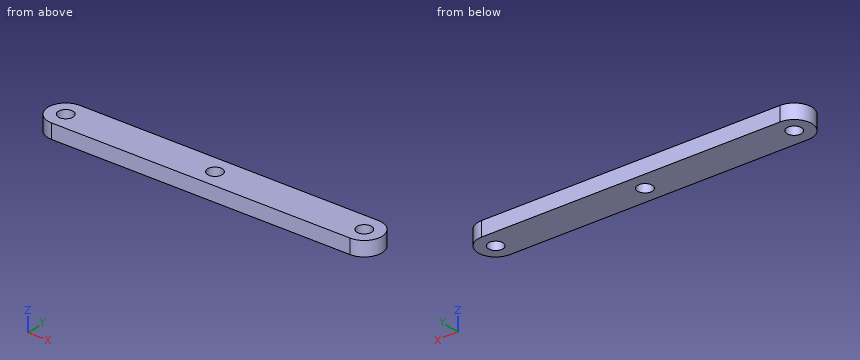
```python
from build123d import *

# Parameters (mm, degrees)
SKETCH1_R           = 2.5
BOSS_EXTRUDE1_DEPTH = 2.5


with BuildPart() as part:
    # Sketch1 → Boss-Extrude1 (new, symmetric)
    with BuildSketch(Plane.XY):
        with BuildLine():
            Line((-50, 6), (50, 6))
            ThreePointArc((50, 6), (56, 0), (50, -6))
            Line((50, -6), (-50, -6))
            ThreePointArc((-50, -6), (-56, 0), (-50, 6))
        make_face()
        with Locations((-50, 0)):
            Circle(SKETCH1_R, mode=Mode.SUBTRACT)
        with Locations((50, 0)):
            Circle(SKETCH1_R, mode=Mode.SUBTRACT)
        Circle(SKETCH1_R, mode=Mode.SUBTRACT)
    extrude(amount=BOSS_EXTRUDE1_DEPTH, both=True)


solid = part.part
```
The listing builds one solid part. Answer for the finished solid, in the listing's coordinates (mm). Give positions to 0.01 mm unless a question says otherwise; leave off trailing zeros. Order: outer loops, then holes, each group sorted by start corner. A loop starts at its lowest first (then second) coordinate and runs counter-clockwise, first axis right, second up. Notation, with made-up numbers: (44.5, 6) -> (75.5, 6) arc R14 ccw to (75.5, 16) -> close; hole circle Ø9 at (38, 57.25). An arc over 180 degrees is marked (long way). Answer as CSV lines item,"result". Start each with the question number.
Q1. A cutting plane is placed at A-A (x = 0). Determine the outline of the cut face in (y, z).
Q2. A cutting plane is placed at B-B (z = -0.15). Determine the outline of the cut face in (x, y).
Q3. Find the intervals of material crossed by L1, parallel to X at y = -0.25, z = 0.6; L2, parallel to X at y = -1.5, z = -0.5; L3, parallel to Y at x = 50, z = -0.8, in increasing order.
Q4. A cutting plane is placed at C-C (y = 0). Determine the outline of the cut face in (x, z), then the cut area to 3 significant figures.
Results found:
1,outline,"(-6, -2.5) -> (-2.5, -2.5) -> (-2.5, 2.5) -> (-6, 2.5) -> close; (2.5, -2.5) -> (6, -2.5) -> (6, 2.5) -> (2.5, 2.5) -> close"
2,outline,"(-50, -6) -> (50, -6) arc R6 ccw to (50, 6) -> (-50, 6) arc R6 ccw to start; hole circle Ø5 at (-50, 0); hole circle Ø5 at (0, 0); hole circle Ø5 at (50, 0)"
3,L1,"-55.99 to -52.49, -47.51 to -2.49, 2.49 to 47.51, 52.49 to 55.99"
3,L2,"-55.81 to -52, -48 to -2, 2 to 48, 52 to 55.81"
3,L3,"-6 to -2.5, 2.5 to 6"
4,outline,"(-56, -2.5) -> (-52.5, -2.5) -> (-52.5, 2.5) -> (-56, 2.5) -> close; (-47.5, -2.5) -> (-2.5, -2.5) -> (-2.5, 2.5) -> (-47.5, 2.5) -> close; (2.5, -2.5) -> (47.5, -2.5) -> (47.5, 2.5) -> (2.5, 2.5) -> close; (52.5, -2.5) -> (56, -2.5) -> (56, 2.5) -> (52.5, 2.5) -> close"
4,area,"485 mm2"
